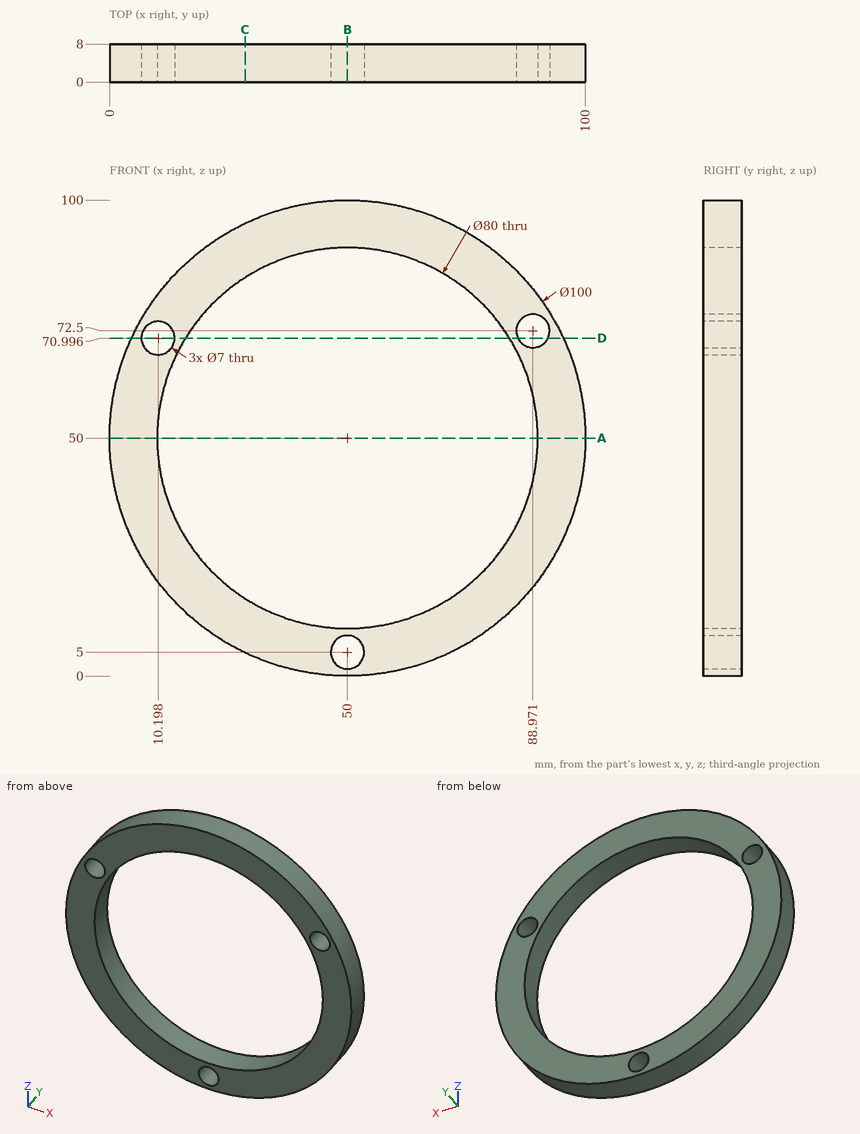
Job drawing, mm, ordinate dimensions from the low corner. One solid piece. Coordinates: 2 decimals unless noted, no trailing zeros. Write each loop counter-clockwise with the first axis right and the second up, starting at its lowest first coordinate (ties: lowest second). Pieces come first, ordered by that corner, then holes. Notation, with made-up numbers: (59, -18.5) -> (73, -18.5) arc R26 cw to (73, -1.5) -> close; hole circle Ø4 at (41, 41.25). An arc over 180 degrees is marked (long way). Use CSV: the item, a comma, the result in double quotes. Start each with the question number.
Item 1: Band-saw the part on B-B, the plane x = 50. Write the cut outline in (y, z), plus the area to 3 significant figures.
Item 2: Band-saw the part on A-A, the plane z = 50. Write the cut outline in (x, y).
Item 3: Band-saw the part on C-C, the plane x = 28.5. Write the cut outline in (y, z).
Item 4: Wall check: probe 1 along X at (y, z) = (1.75, 49.5); probe 2 along X at (y, z) = (6.5, 72.5); probe 3 along Z at (x, y) = (52, 7.5). Give the ranges that are in metal, low to high.
Item 5: Band-saw the part on D-D, the plane z = 71. Write the cut outline in (x, y) (1 decimal).
Item 6: Drop flat-ended pins along their axis: P1, Ø4, axis at x = 18, y = 4, coming from the +Z side; P2, Ø2, axis at y = 5, z = 38, coming from the -X side (1 decimal); P3, Ø2, axis at x = 19.5, y = 6.5, coming from the -Z side. Give the stop position or say it passes through.
Response values:
1,outline,"(0, 0) -> (8, 0) -> (8, 1.5) -> (0, 1.5) -> close; (0, 8.5) -> (8, 8.5) -> (8, 10) -> (0, 10) -> close; (0, 90) -> (8, 90) -> (8, 100) -> (0, 100) -> close"
1,area,"104 mm2"
2,outline,"(0, 0) -> (10, 0) -> (10, 8) -> (0, 8) -> close; (90, 0) -> (100, 0) -> (100, 8) -> (90, 8) -> close"
3,outline,"(0, 4.86) -> (8, 4.86) -> (8, 16.27) -> (0, 16.27) -> close; (0, 83.73) -> (8, 83.73) -> (8, 95.14) -> (0, 95.14) -> close"
4,probe 1,"x = 0 to 10, 90 to 100"
4,probe 2,"x = 5.35 to 7.04, 13.36 to 16.93, 83.07 to 85.47, 92.47 to 94.65"
4,probe 3,"z = 0.04 to 2.13, 7.87 to 10.05, 89.95 to 99.96"
5,outline,"(4.6, 0) -> (6.7, 0) -> (6.7, 8) -> (4.6, 8) -> close; (13.7, 0) -> (16, 0) -> (16, 8) -> (13.7, 8) -> close; (84, 0) -> (85.8, 0) -> (85.8, 8) -> (84, 8) -> close; (92.1, 0) -> (95.4, 0) -> (95.4, 8) -> (92.1, 8) -> close"
6,P1,"stops at z = 90"
6,P2,"stops at x = 1.2"
6,P3,"stops at z = 9.63"
